Model file for the job. Use its own axes, mm. A direction names the side the tool comes from. Round coordinates to 2 decimals unless told otherwise and drop trailing zeros. Loops run counter-clockwise (first coordinate to the right, second up) from the corner with the lowest first, then second, coordinate; pieces in that order, holes last. Notation, with made-up numbers: (22, 85.25) -> (72, 85.25) arc R31 ccw to (72, 124.25) -> close; hole circle Ø9 at (-29, 30). An arc over 180 degrees is marked (long way). Use a Markdown table: item, result.
from build123d import *

# Parameters (mm, degrees)
SKETCH1_R           = 2
SKETCH1_R_2         = 1.25
SKETCH1_R_3         = 11
BOSS_EXTRUDE1_DEPTH = 3
FILLET1_R           = 3
FILLET2_R           = 3
FILLET3_R           = 3
FILLET4_R           = 3
FILLET5_R           = 3
FILLET7_R           = 3
FILLET8_R           = 2
FILLET9_R           = 2


with BuildPart() as part:
    # Sketch1 → Boss-Extrude1 (new body)
    with BuildSketch(Plane(origin=(0, 0, 0), x_dir=(1, 0, 0), z_dir=(0, 1, 0))):
        Polygon((0, 111.61362417), (-32.5, 111.61362417), (-32.5, 56.61362417), (-22.5, 56.61362417), (-22.5, -58.38637583), (0, -58.38637583), (22.5, -58.38637583), (22.5, 56.61362417), (32.5, 56.61362417), (32.5, 111.61362417), align=None)
        with Locations(Location((0, 91.61362417, 0), (0, 0, 270))):
            Circle(SKETCH1_R, mode=Mode.SUBTRACT)
        with Locations(Location((0, 66.61362417, 0), (0, 0, 270))):
            Circle(SKETCH1_R, mode=Mode.SUBTRACT)
        with Locations(Location((-15.5, -20.454039675, 0), (0, 0, 270))):
            Circle(SKETCH1_R_2, mode=Mode.SUBTRACT)
        with Locations(Location((-15.5, -51.454039675, 0), (0, 0, 270))):
            Circle(SKETCH1_R_2, mode=Mode.SUBTRACT)
        with Locations(Location((15.5, -51.454039675, 0), (0, 0, 270))):
            Circle(SKETCH1_R_2, mode=Mode.SUBTRACT)
        with Locations(Location((15.5, -20.454039675, 0), (0, 0, 270))):
            Circle(SKETCH1_R_2, mode=Mode.SUBTRACT)
        with Locations(Location((0, -35.954039675, 0), (0, 0, 270))):
            Circle(SKETCH1_R_3, mode=Mode.SUBTRACT)
        with Locations(Location((0, 11.61362417, 0), (0, 0, 270))):
            Circle(SKETCH1_R, mode=Mode.SUBTRACT)
    extrude(amount=BOSS_EXTRUDE1_DEPTH)

    # Fillet1
    fillet1_edges = [part.edges().sort_by_distance(p)[0] for p in [
        (32.5, 1.5, -111.61362417),
    ]]
    fillet(fillet1_edges, radius=FILLET1_R)

    # Fillet2
    fillet2_edges = [part.edges().sort_by_distance(p)[0] for p in [
        (-32.5, 1.5, -111.61362417),
    ]]
    fillet(fillet2_edges, radius=FILLET2_R)

    # Fillet3
    fillet3_edges = [part.edges().sort_by_distance(p)[0] for p in [
        (-32.5, 1.5, -56.61362417),
    ]]
    fillet(fillet3_edges, radius=FILLET3_R)

    # Fillet4
    fillet4_edges = [part.edges().sort_by_distance(p)[0] for p in [
        (32.5, 1.5, -56.61362417),
    ]]
    fillet(fillet4_edges, radius=FILLET4_R)

    # Fillet5
    fillet5_edges = [part.edges().sort_by_distance(p)[0] for p in [
        (22.5, 1.5, 58.38637583),
    ]]
    fillet(fillet5_edges, radius=FILLET5_R)

    # Fillet7
    fillet7_edges = [part.edges().sort_by_distance(p)[0] for p in [
        (-22.5, 1.5, 58.38637583),
    ]]
    fillet(fillet7_edges, radius=FILLET7_R)

    # Fillet8
    fillet8_edges = [part.edges().sort_by_distance(p)[0] for p in [
        (-22.5, 1.5, -56.61362417),
    ]]
    fillet(fillet8_edges, radius=FILLET8_R)

    # Fillet9
    fillet9_edges = [part.edges().sort_by_distance(p)[0] for p in [
        (22.5, 1.5, -56.61362417),
    ]]
    fillet(fillet9_edges, radius=FILLET9_R)


solid = part.part
Q1. Tool access for faces 4 (the face through (22.5, 1, 1)), 5 (the face through (-22.5, 1, 0)), 6 (the face through (31.598, 1.521, -110.758)): list every direction of +Z, -Z, +X, -X, +Y, -Y with a clear straight run to the whole face (end or side of a thin tool).
Results list:
| item | result |
|---|---|
| face 4 | +Z, +X, +Y, -Y |
| face 5 | +Z, -X, +Y, -Y |
| face 6 | -Z, +X, +Y, -Y |
Q2. Drill centre lines: L1, parallel to Z at x = 1.5, y = 0.45; L2, parallel to Z at x = 15, y = 0.3; L3, parallel to X at y = 0.35, z = 33.5. Where is each one in solid material? Low to high. Write a range as from..to.
Results list:
| item | result |
|---|---|
| L1 | z = -111.61..-92.94, -90.29..-67.94, -65.29..-12.94, -10.29..25.06, 46.85..58.39 |
| L2 | z = -111.61..19.31, 21.6..50.31, 52.6..58.39 |
| L3 | x = -22.5..-10.72, 10.72..22.5 |
Q3. Pull direction Z, two halves, no side cores. Call faces 1 (the face through (-4.213, 1.479, 46.115)), 2 (the face through (0, 1, -111.614)), 3 (the face through (-27, 1, -56.614)): released by +Z, released by -Z, zero draft, split by the parting line, or undercut.
Results list:
| item | result |
|---|---|
| face 1 | undercut |
| face 2 | released by -Z |
| face 3 | released by +Z |
Q4. Band-saw the part on D-D, the plane x = 8. Give the cut face in (y, z).
Results list:
| item | result |
|---|---|
| outline | (0, -111.61) -> (3, -111.61) -> (3, 28.4) -> (0, 28.4) -> close; (0, 43.5) -> (3, 43.5) -> (3, 58.39) -> (0, 58.39) -> close |
Q5. Flat gauge pins, fed straight in: pin 1 (3 mm diameter, centred on x = -15.5, z = 51.45, fed in from -Y); pin 2 (13 mm diameter, centred on x = 0, z = 35.95, fed in from +Y); pin 3 (1.5 mm diameter, centred on x = -28, y = 1, fed in from +Z). Where does each tip first touch, or does it go through?
Results list:
| item | result |
|---|---|
| pin 1 | stops at y = 0 |
| pin 2 | passes through |
| pin 3 | stops at z = -56.61 |
Q6. Band-saw the part on A-A, the plane x = 0. Give the cut face in (y, z), plus the area to 3 significant figures.
Results list:
| item | result |
|---|---|
| outline | (0, -111.61) -> (3, -111.61) -> (3, -93.61) -> (0, -93.61) -> close; (0, -89.61) -> (3, -89.61) -> (3, -68.61) -> (0, -68.61) -> close; (0, -64.61) -> (3, -64.61) -> (3, -13.61) -> (0, -13.61) -> close; (0, -9.61) -> (3, -9.61) -> (3, 24.95) -> (0, 24.95) -> close; (0, 46.95) -> (3, 46.95) -> (3, 58.39) -> (0, 58.39) -> close |
| area | 408 mm² |
Q7. Band-saw the part on B-B, the plane y = 2. Give the number of separate pieces and of enclosed holes in the cut face, plus the area to 3 significant figures.
Results list:
| item | result |
|---|---|
| separate pieces | 1 |
| enclosed holes | 8 |
| area | 8,300 mm² |
Q8. Band-saw the part on C-C, the plane z = 32. Give the cut face in (x, y).
Results list:
| item | result |
|---|---|
| outline | (-22.5, 0) -> (-10.26, 0) -> (-10.26, 3) -> (-22.5, 3) -> close; (10.26, 0) -> (22.5, 0) -> (22.5, 3) -> (10.26, 3) -> close |
